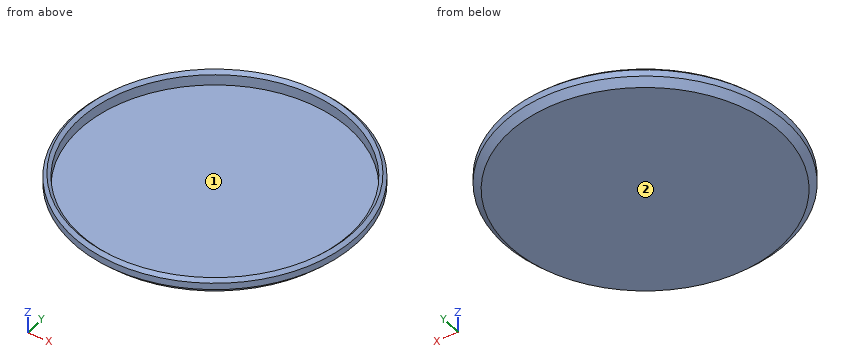
from build123d import *

# Parameters (mm, degrees)
F0_R     = 40.5
F1_DEPTH = 0.8
F0_R_2   = 42.5
F2_DEPTH = 5
F3_SIZE  = 2
F4_SIZE  = 0.99999


# Not quite as in the source:
# - a fillet or chamfer is up to 0.001 mm smaller than in the source, because OpenCascade refuses the exact size


with BuildPart() as f1:
    # F0 (on Top) → F1 (new body)
    with BuildSketch(Plane.XY):
        Circle(F0_R)
    extrude(amount=F1_DEPTH)

    # F0 (on Top) → F2 (join)
    with BuildSketch(Plane.XY):
        Circle(F0_R_2)
        Circle(F0_R, mode=Mode.SUBTRACT)
    extrude(amount=F2_DEPTH)

    # F3
    f3_edges = [f1.edges().sort_by_distance(p)[0] for p in [
        (-42.5, 0, 0),
    ]]
    chamfer(f3_edges, length=F3_SIZE)

    # F4 (size 1 in the source; OpenCascade refuses exactly that, so slightly less here)
    f4_edges = [f1.edges().sort_by_distance(p)[0] for p in [
        (-40.5, 0, 5),
        (-42.5, 0, 5),
    ]]
    chamfer(f4_edges, length=F4_SIZE)


solid = f1.part
Can you work these out from the model? Positions are in its coordinate system, mm. Face numbers are marked on the shaded views. Round coordinates to 2 decimals unless told otherwise and drop trailing zeros. Write each question's results on one line, items separated by ' | '. Start each with the question number.
Item 1: Will these pins go through, and if not, where does the flat tip stop? pin 1 (3 mm diameter, centred on y = 28.5, z = 1.5, fed in from -X); pin 2 (1 mm diameter, centred on x = 24.5, z = 3.5, fed in from +Y); pin 3 (1.5 mm diameter, centred on x = -2, z = 1, fed in from +Y).
Item 2: Thinking about a two-plate mould opening in X: for the marked faces 1 and 2, which applies, +X half, -X half, draft (parallel to the pull), parting line (faces both ways), or undercut?
Item 3: Please list where these lines run through material, in increasing order: L1, parallel to Y at x = 0, z = 3.35; L2, parallel to Z at x = -17.5, y = -1; L3, parallel to X at y = 34.5, z = 2.9.
Results:
1) pin 1: stops at x = -32.75 | pin 2: stops at y = 35.07 | pin 3: stops at y = 42.2
2) face 1: undercut | face 2: draft
3) L1: y = -42.5 to -40.5, 40.5 to 42.5 | L2: z = 0 to 0.8 | L3: x = -24.82 to -21.21, 21.21 to 24.82
